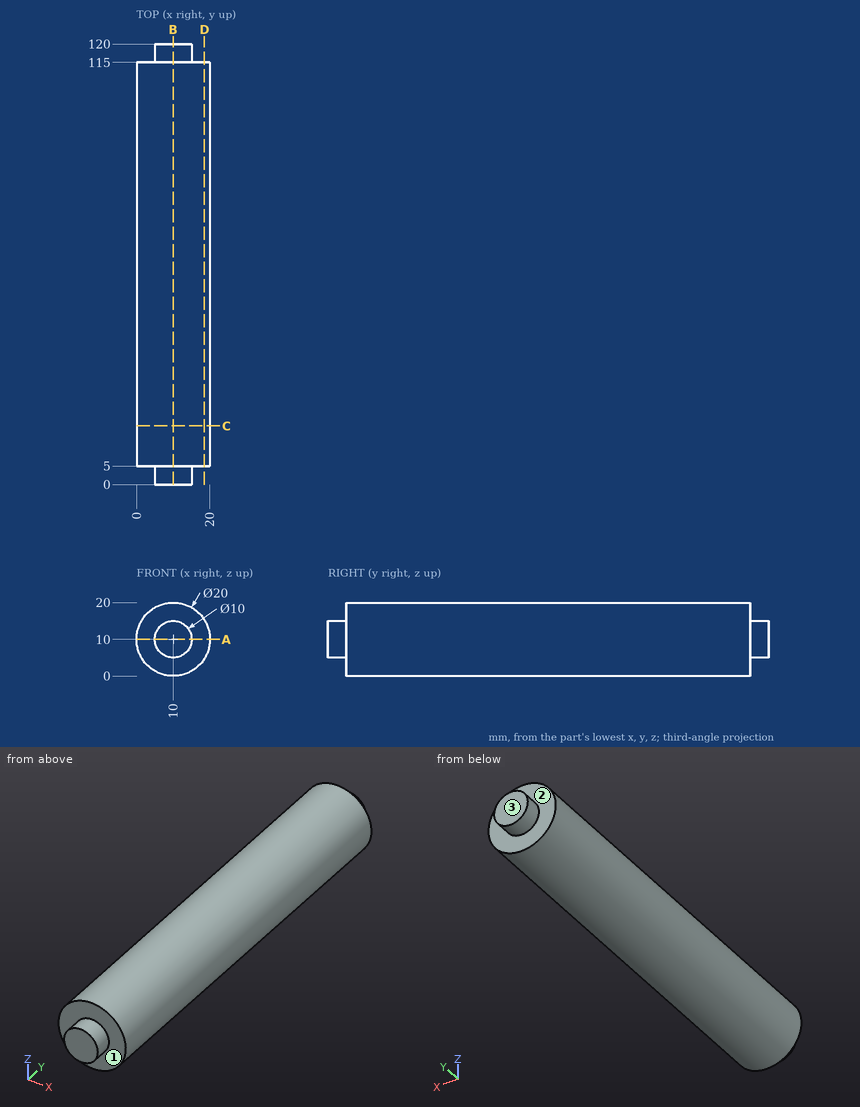
Geometry: see drawing. Coordinates: mm, zero at the bounding-box minimum. A direction names the side the tool comes from. Give positions to 0.01 mm unless a question says otherwise; leave off trailing zeros. Order: outer loops, then holes, each group sorted by start corner. A loop starts at its lowest first (then second) coordinate and runs counter-clockwise, first axis right, second up. Notation, with made-up numbers: M 67.5,11.25 L 125.5,11.25 A18 ccw 125.5,43.25 Z; hole C 58,77 d3. An arc over 180 degrees is marked long. Answer as CSV lines item,"result". Start each with the question number.
1) Cut plane B-B (x = 10). Output: boundary loops of the cut face in (y, z), then the cut area to 3 significant figures.
2) Line query: line 1 (Y direction, x = 1, z = 14.25); line 2 (Z direction, x = 9.75, y = 29); line 3 (X direction, y = 12, z = 9.5). Output: solid intervals per line, ascending. Write a range as from..to.
3) Cut plane C-C (y = 16). Output: boundary loops of the cut face in (x, z).
4) Cut plane D-D (x = 18.5). Output: boundary loops of the cut face in (y, z).
5) Cut plane A-A (z = 10). Output: boundary loops of the cut face in (x, y).
6) First-contact query: P1, Ø1.5, axis at x = 3, z = 14.5, coming from the -Y side; P2, Ø3, axis at x = 17, y = 33.5, coming from the -Z side; P3, Ø2, axis at y = 74, z = 14, coming from the +X side. Flat tips, straight axial feed; report the tip coordinate or a pass-through.
7) Set-up query: the marked faces 1, 2 and 3. Return all of +Z, -Z, +X, -X, +Y, -Y with unobstructed straight access to the full face (end or side cutting, diameter ignored); none if empty.
Findings below:
1,outline,"M 0,5 L 5,5 L 5,0 L 115,0 L 115,5 L 120,5 L 120,15 L 115,15 L 115,20 L 5,20 L 5,15 L 0,15 Z"
1,area,"2,300 mm²"
2,line 1,"y = 5..115"
2,line 2,"z = 0..20"
2,line 3,"x = 0.01..19.99"
3,outline,"C 10,10 d20"
4,outline,"M 5,4.73 L 115,4.73 L 115,15.27 L 5,15.27 Z"
5,outline,"M 0,5 L 5,5 L 5,0 L 15,0 L 15,5 L 20,5 L 20,115 L 15,115 L 15,120 L 5,120 L 5,115 L 0,115 Z"
6,P1,"stops at y = 5"
6,P2,"stops at z = 1.65"
6,P3,"stops at x = 19.54"
7,face 1,"-Y"
7,face 2,"+Y"
7,face 3,"+Z, -Z, +X, -X, +Y"
